```python
from build123d import *

# Parameters (mm, degrees)
F0_W     = 50.8
F0_H     = 61.80582
F0_W_2   = 44.45
F0_H_2   = 57.15762
F1_DEPTH = 1.5875
F2_R     = 0.79375
F3_DEPTH = 0.79375


with BuildPart() as f1:
    # F0 (on Front) → F1 (new body)
    with BuildSketch(Plane.XZ):
        Rectangle(F0_W, F0_H)
        with Locations((0, 0.8509)):
            Rectangle(F0_W_2, F0_H_2, mode=Mode.SUBTRACT)
    extrude(amount=F1_DEPTH)

    # F2 (on face) → F3 (cut)
    with BuildSketch(Plane(origin=(0, 0, 0), x_dir=(-1, 0, 0), z_dir=(0, 1, 0))):
        with Locations((-23.8125, 29.31541)):
            Circle(F2_R)
        with Locations((-23.8125, -29.31541)):
            Circle(F2_R)
        with Locations((23.8125, -29.31541)):
            Circle(F2_R)
        with Locations((23.8125, 29.31541)):
            Circle(F2_R)
    extrude(amount=-F3_DEPTH, mode=Mode.SUBTRACT)


solid = f1.part
```
Verification items for the finished model (mm, model axes). A direction names the side the tool comes from. Give positions to 0.01 mm unless a question says otherwise; leave off trailing zeros. Order: outer loops, then holes, each group sorted by start corner. A loop starts at its lowest first (then second) coordinate and runs counter-clockwise, first axis right, second up. Notation, with made-up numbers: M -11,70.25 L 46,70.25 A16 cw 46,85.25 Z; hole C 81,-13 d3. An arc over 180 degrees is marked long. Answer in a Markdown table with one row per item. Add a question column.
Item 1: Scan lines: probe 1 along X at (y, z) = (-0.1, 9) (3 decimals); probe 2 along Z at (x, y) = (14.5, -0.5). Record each from-to range of solid material in increasing order. Write a range as from..to.
Item 2: Section check B-B, the plane x = -5. Enter the section's corners in (y, z).
Item 3: Gauge pin test, flat ends, axial feed: pin 1 (1.7 mm diameter, centred on x = 24, z = 29.5, fed in from +Y); pin 2 (1.4 mm diameter, centred on x = 23.81, z = 29.32, fed in from +Y). Record the tip position at first contact, or that the pin passes through.
Item 4: Tool access check on faces 5 (the cylindrical face through (23.08, -0.39, 29.01)), 6 (the flat face through (0, -1, -30.903)), 7 (the flat face through (22.225, -1, 0)). Record the directions out of +Z, -Z, +X, -X, +Y, -Y that give a thin tool (end or side, any length) a straight path to the whole face; none if there is none.
Item 5: Section check C-C, the plane y = -1.2. Enter the section's corners in (x, z) (3 decimals).
Item 6: Mould release check, pull along X, two halves, no side actions. Record for faces 1 (the flat face through (24, -0.794, -29)), 2 (the flat face through (-23, 0, 0)), 3 (the flat face through (-25.4, -1, 0)), 4 (the flat face through (25.4, -1, 0)): released by +X, released by -X, zero draft, split by the parting line, or undercut.
Item 7: Section check A-A, the plane z = 17. Enter the section's corners in (x, y) (1 decimal), and give its area (3 significant figures).
Filled sheet:
| question | item | result |
|---|---|---|
| 1 | probe 1 | x = -25.4..-22.225, 22.225..25.4 |
| 1 | probe 2 | z = -30.9..-27.73, 29.43..30.9 |
| 2 | outline | M -1.59,-30.9 L 0,-30.9 L 0,-27.73 L -1.59,-27.73 Z; M -1.59,29.43 L 0,29.43 L 0,30.9 L -1.59,30.9 Z |
| 3 | pin 1 | stops at y = 0 |
| 3 | pin 2 | stops at y = -0.79 |
| 4 | face 5 | +Y |
| 4 | face 6 | -Z, +X, -X, +Y, -Y |
| 4 | face 7 | +Y, -Y |
| 5 | outline | M -25.4,-30.903 L 25.4,-30.903 L 25.4,30.903 L -25.4,30.903 Z; hole M -22.225,-27.728 L 22.225,-27.728 L 22.225,29.43 L -22.225,29.43 Z |
| 6 | face 1 | undercut |
| 6 | face 2 | zero draft |
| 6 | face 3 | released by -X |
| 6 | face 4 | released by +X |
| 7 | outline | M -25.4,-1.6 L -22.2,-1.6 L -22.2,0 L -25.4,0 Z; M 22.2,-1.6 L 25.4,-1.6 L 25.4,0 L 22.2,0 Z |
| 7 | area | 10.1 mm^2 |
